CAD build for the part. Positions are in the model's coordinates, mm. Round coordinates to 2 decimals unless told otherwise and drop trailing zeros. Loops run counter-clockwise (first coordinate to the right, second up) from the corner with the lowest first, then second, coordinate; pieces in that order, holes last.
```python
from build123d import *

# Parameters (mm, degrees)
SKETCH2_R           = 3.175
SKETCH2_R_2         = 4.7625
SKETCH2_R_3         = 4
SKETCH2_W           = 11.850089675
SKETCH2_H           = 89.916
SKETCH2_W_2         = 60
SKETCH2_H_2         = 10
SKETCH2_W_3         = 10.16
SKETCH2_H_3         = 63.685061478
SKETCH2_H_4         = 63.685061479
SKETCH2_H_5         = 76.2
BOSS_EXTRUDE1_DEPTH = 10.16
SKETCH4_W           = 351.675616699
SKETCH4_H           = 10.16
BOSS_EXTRUDE2_DEPTH = 60.261226


with BuildPart() as part:
    # Sketch2 → Boss-Extrude1 (new body)
    with BuildSketch(Plane.XY):
        with BuildLine():
            Line((-408.921789204, 152.75736057), (-459.721789204, 152.75736057))
            Line((-459.721789204, 152.75736057), (-459.721789204, -230.782639429))
            ThreePointArc((-459.721789204, -230.782639429), (-437.403325931, -284.664176156), (-383.521789204, -306.982639429))
            Line((-383.521789204, -306.982639429), (-303.52, -306.982639429))
            Line((-303.52, -306.982639429), (-270.8, -306.982639429))
            Line((-270.8, -306.982639429), (-270.8, -317.142639429))
            Line((-270.8, -317.142639429), (-220, -317.142639429))
            Line((-220, -317.142639429), (-220, -306.982639429))
            Line((-220, -306.982639429), (-55.8292, -306.982639429))
            Line((-55.8292, -306.982639429), (-55.8292, -317.142639429))
            Line((-55.8292, -317.142639429), (55.8292, -317.142639429))
            Line((55.8292, -317.142639429), (55.8292, -306.982639429))
            Line((55.8292, -306.982639429), (220, -306.982639429))
            Line((220, -306.982639429), (220, -317.142639429))
            Line((220, -317.142639429), (270.8, -317.142639429))
            Line((270.8, -317.142639429), (270.8, -306.982639429))
            Line((270.8, -306.982639429), (303.52, -306.982639429))
            Line((303.52, -306.982639429), (383.521789204, -306.982639429))
            ThreePointArc((383.521789204, -306.982639429), (437.403325931, -284.664176156), (459.721789204, -230.782639429))
            Line((459.721789204, -230.782639429), (459.721789204, 152.75736057))
            Line((459.721789204, 152.75736057), (408.921789204, 152.75736057))
            Line((408.921789204, 152.75736057), (408.921789204, 142.616356263))
            Line((408.921789204, 142.616356263), (332.721789204, 142.616356263))
            Line((332.721789204, 142.616356263), (332.721789204, 152.75736057))
            Line((332.721789204, 152.75736057), (135.250547773, 152.75736057))
            Line((135.250547773, 152.75736057), (102.394461083, 316.728644457))
            Line((102.394461083, 316.728644457), (-102.394461083, 316.728644457))
            Line((-102.394461083, 316.728644457), (-135.250547773, 152.75736057))
            Line((-135.250547773, 152.75736057), (-332.100796745, 152.75736057))
            Line((-332.100796745, 152.75736057), (-332.100796745, 142.616356263))
            Line((-332.100796745, 142.616356263), (-408.300796745, 142.616356263))
            Line((-408.300796745, 142.616356263), (-408.921789204, 152.75736057))
        make_face()
        with Locations((336.550272189, -94.687385458)):
            Circle(SKETCH2_R, mode=Mode.SUBTRACT)
        with Locations((378.573819589, -5.78737531)):
            Circle(SKETCH2_R, mode=Mode.SUBTRACT)
        with Locations((336.550272189, -5.787385458)):
            Circle(SKETCH2_R, mode=Mode.SUBTRACT)
        with Locations((336.550272189, 83.112614542)):
            Circle(SKETCH2_R, mode=Mode.SUBTRACT)
        with Locations((412.750272189, 83.112614542)):
            Circle(SKETCH2_R, mode=Mode.SUBTRACT)
        with Locations((-412.75027219, 83.112614542)):
            Circle(SKETCH2_R, mode=Mode.SUBTRACT)
        with Locations((-336.55027219, 83.112614542)):
            Circle(SKETCH2_R, mode=Mode.SUBTRACT)
        with Locations((-336.55027219, -5.787385458)):
            Circle(SKETCH2_R, mode=Mode.SUBTRACT)
        with Locations((-378.573819589, -5.78737531)):
            Circle(SKETCH2_R, mode=Mode.SUBTRACT)
        with Locations((-336.55027219, -94.687385458)):
            Circle(SKETCH2_R, mode=Mode.SUBTRACT)
        with Locations((172.2755, 127.35736057)):
            Circle(SKETCH2_R_2, mode=Mode.SUBTRACT)
        with Locations((172.2755, 25.75736057)):
            Circle(SKETCH2_R_2, mode=Mode.SUBTRACT)
        with Locations((81.7245, 25.75736057)):
            Circle(SKETCH2_R_2, mode=Mode.SUBTRACT)
        with Locations((81.7245, 127.35736057)):
            Circle(SKETCH2_R_2, mode=Mode.SUBTRACT)
        with Locations((-81.7245, 25.75736057)):
            Circle(SKETCH2_R_2, mode=Mode.SUBTRACT)
        with Locations((-81.7245, 127.35736057)):
            Circle(SKETCH2_R_2, mode=Mode.SUBTRACT)
        with Locations((-172.2755, 127.35736057)):
            Circle(SKETCH2_R_2, mode=Mode.SUBTRACT)
        with Locations((-172.2755, 25.75736057)):
            Circle(SKETCH2_R_2, mode=Mode.SUBTRACT)
        with Locations((0, -78.38263943)):
            Circle(SKETCH2_R, mode=Mode.SUBTRACT)
        with Locations((95.25, -84.73263943)):
            Circle(SKETCH2_R_2, mode=Mode.SUBTRACT)
        with Locations((-172.69, -239.442639429)):
            Circle(SKETCH2_R_3, mode=Mode.SUBTRACT)
        with Locations((-117.38, -239.442639429)):
            Circle(SKETCH2_R_3, mode=Mode.SUBTRACT)
        with Locations((-117.38, -269.442639429)):
            Circle(SKETCH2_R_3, mode=Mode.SUBTRACT)
        with Locations((-172.69, -269.442639429)):
            Circle(SKETCH2_R_3, mode=Mode.SUBTRACT)
        with Locations((311.557332494, 7.72336057)):
            Rectangle(SKETCH2_W, SKETCH2_H, mode=Mode.SUBTRACT)
        with Locations((311.557332494, -172.10863943)):
            Rectangle(SKETCH2_W, SKETCH2_H, mode=Mode.SUBTRACT)
        with Locations((-365.16, -74.446988355)):
            Rectangle(SKETCH2_W_2, SKETCH2_H_2, mode=Mode.SUBTRACT)
        Polygon((-270.16, -79.446988355), (-210.16, -79.446988355), (-210.16, -85.16237531), (-200, -85.16237531), (-200, -8.96237531), (-210.16, -8.96237531), (-210.16, -69.446988355), (-270.16, -69.446988355), align=None, mode=Mode.SUBTRACT)
        with Locations((195.58, -147.752560311)):
            Rectangle(SKETCH2_W_3, SKETCH2_H_3, mode=Mode.SUBTRACT)
        with Locations((195.58, -20.382437355)):
            Rectangle(SKETCH2_W_3, SKETCH2_H_4, mode=Mode.SUBTRACT)
        with Locations((195.58, 106.97026018)):
            Rectangle(SKETCH2_W_3, SKETCH2_H_4, mode=Mode.SUBTRACT)
        with Locations((-205.08, -256.782661115)):
            Rectangle(SKETCH2_W_3, SKETCH2_H_5, mode=Mode.SUBTRACT)
        with Locations((-240.16, -186.254154613)):
            Rectangle(SKETCH2_W_2, SKETCH2_H_2, mode=Mode.SUBTRACT)
        with Locations((-365.16, -186.254154613)):
            Rectangle(SKETCH2_W_2, SKETCH2_H_2, mode=Mode.SUBTRACT)
        with Locations((-311.557332494, -172.10863943)):
            Rectangle(SKETCH2_W, SKETCH2_H, mode=Mode.SUBTRACT)
        with Locations((-84.92, -256.782661115)):
            Rectangle(SKETCH2_W_3, SKETCH2_H_5, mode=Mode.SUBTRACT)
        with Locations((-84.92, -47.06237531)):
            Rectangle(SKETCH2_W_3, SKETCH2_H_5, mode=Mode.SUBTRACT)
        with Locations((-311.557332494, 7.72336057)):
            Rectangle(SKETCH2_W, SKETCH2_H, mode=Mode.SUBTRACT)
        with BuildLine():
            Line((-108.5, -221.170881029), (-138.5, -221.170881029))
            ThreePointArc((-138.5, -221.170881029), (-152, -207.670881029), (-138.5, -194.170881029))
            Line((-138.5, -194.170881029), (-108.5, -194.170881029))
            ThreePointArc((-108.5, -194.170881029), (-95, -207.670881029), (-108.5, -221.170881029))
        make_face(mode=Mode.SUBTRACT)
    extrude(amount=-BOSS_EXTRUDE1_DEPTH)

    # Sketch4 → Boss-Extrude2 (add)
    with BuildSketch(Plane(origin=(0, 152.75736057, 0), x_dir=(1, 0, 0), z_dir=(0, 1, 0))):
        with Locations((-283.883980855, 5.08)):
            Rectangle(SKETCH4_W, SKETCH4_H)
    extrude(amount=BOSS_EXTRUDE2_DEPTH)


solid = part.part
```
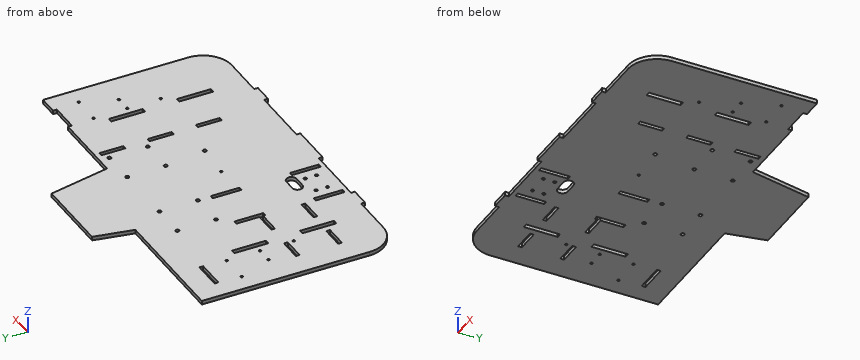
Item 1: Cut at B-B, the plane z = -3. State how many separate pieces and enclosed holes the cut face has, plus the area to 3 significant figures.
Answers follow:
separate pieces: 1
enclosed holes: 40
area: 465,000 mm2
Item 2: Flat gauge pins, fed straight in: P1, Ø1, axis at x = 188, y = -1.5, coming from the +Z side; P2, Ø5, axis at x = 311, z = -7, coming from the +Y side; P3, Ø5, axis at x = -352, z = -6, coming from the +Y side; P4, Ø3, axis at x = 311.5, z = -5.5, coming from the -Y side. Where does each tip first touch, or does it go through?
Answers follow:
P1: stops at z = 0
P2: stops at y = 152.76
P3: stops at y = 213.02
P4: stops at y = -306.98
Item 3: Probe line 1 (X direction, y = 1.5, z = -0.75); line 2 (Y direction, x = -220.5, z = -0.5); line 3 (X direction, y = -79.5, z = -5.25). List the from-to ranges inside material, lowest first.
Answers follow:
line 1: x = -459.72 to -317.48, -305.63 to 190.5, 200.66 to 305.63, 317.48 to 459.72
line 2: y = -317.14 to -191.25, -181.25 to -79.45, -69.45 to 213.02
line 3: x = -459.72 to -210.16, -200 to -90, -79.84 to -2.97, 2.97 to 459.72
Item 4: Cut at A-A, the plane x = -294.5. Give the cut face in (y, z), plus the area to 3 significant figures.
Answers follow:
outline: (-306.98, -10.16) - (213.02, -10.16) - (213.02, 0) - (-306.98, 0) - close
area: 5,280 mm2
